Build history of the part. All positions in model axes, mm. A direction names the side the tool comes from. Round coordinates to 2 decimals unless told otherwise and drop trailing zeros. Order: outer loops, then holes, each group sorted by start corner. A loop starts at its lowest first (then second) coordinate and runs counter-clockwise, first axis right, second up. Notation, with made-up numbers: M 80.25,29 L 117.25,29 A14 cw 117.25,42 Z; hole C 61.25,12 d6. An arc over 180 degrees is marked long. One line per item, written item: value. Start each with the question number.
Item 1: Two-plate mould, pull along Z, no slides. Class faces 1 (the flat face through (-1, 15, -24)), 2 (the flat face through (-45, 14, 0.75)), 3 (the flat face through (49, 15, 0)), 4 (the flat face through (-1, 15, 24)): +Z half, -Z half, draft (parallel to the pull), parting line (faces both ways), or undercut.
Item 2: Probe L1, parallel to Z at x = 44, y = 13.25; L2, parallel to X at y = 9.25, z = 20; L3, parallel to X at y = 24, z = 0. List the from-to ranges inside material, lowest first.
Item 3: Tool access for faces 5 (the flat face through (-1, 16, 22.5)), 6 (the flat face through (-49, 15, 0)): list every direction of +Z, -Z, +X, -X, +Y, -Y with a clear straight run to the whole face (end or side of a thin tool).
Item 4: Band-saw the part on C-C, the plane x = -1. Write the cut outline in (y, z).
Item 5: Pin check, flat tips, straight feed: pin 1 (13.5 mm diameter, centred on x = 18.5, z = 1, fed in from +Y); pin 2 (1 mm diameter, centred on x = -10.5, z = -0.5, fed in from -Y); pin 3 (0.8 mm diameter, centred on x = 21, z = -21, fed in from +Y). Stop position of each tip, or through.
Item 6: Band-saw the part on A-A, the plane z = 19. Write the cut outline in (x, y).
```python
from build123d import *

# Parameters (mm, degrees)
SKETCH1_W           = 98
SKETCH1_H           = 48
BOSS_EXTRUDE1_DEPTH = 30
SHELL1_T            = -1.5
SKETCH2_W           = 1.5
SKETCH2_H           = 5
SKETCH2_W_2         = 5
SKETCH2_H_2         = 1.5
BOSS_EXTRUDE2_DEPTH = 25.5


with BuildPart() as part:
    # Sketch1 → Boss-Extrude1 (new body)
    with BuildSketch(Plane(origin=(0, 0, 0), x_dir=(1, 0, 0), z_dir=(0, 1, 0))):
        Rectangle(SKETCH1_W, SKETCH1_H)
    extrude(amount=BOSS_EXTRUDE1_DEPTH)

    # Shell1
    shell1_openings = [part.faces().sort_by_distance(p)[0] for p in [
        (0, 30, 0),
    ]]
    offset(amount=SHELL1_T, openings=shell1_openings, kind=Kind.INTERSECTION)

    # Sketch2 → Boss-Extrude2 (add)
    with BuildSketch(Plane(origin=(0, 1.5, 0), x_dir=(1, 0, 0), z_dir=(0, 1, 0))):
        with Locations((-20.75, 20)):
            Rectangle(SKETCH2_W, SKETCH2_H)
        with Locations((20.75, 20)):
            Rectangle(SKETCH2_W, SKETCH2_H)
        with Locations((20.75, -20)):
            Rectangle(SKETCH2_W, SKETCH2_H)
        with Locations((-20.75, -20)):
            Rectangle(SKETCH2_W, SKETCH2_H)
        with Locations((45, 0)):
            Rectangle(SKETCH2_W_2, SKETCH2_H_2)
        with Locations((-45, 0)):
            Rectangle(SKETCH2_W_2, SKETCH2_H_2)
    extrude(amount=BOSS_EXTRUDE2_DEPTH)


solid = part.part
```
Output:
1. face 1: -Z half
1. face 2: undercut
1. face 3: draft
1. face 4: +Z half
2. L1: z = -24 to -22.5, -0.75 to 0.75, 22.5 to 24
2. L2: x = -49 to -47.5, -21.5 to -20, 20 to 21.5, 47.5 to 49
2. L3: x = -49 to -42.5, 42.5 to 49
3. face 5: +Y
3. face 6: +Z, -Z, -X, +Y, -Y
4. outline: M 0,-24 L 30,-24 L 30,-22.5 L 1.5,-22.5 L 1.5,22.5 L 30,22.5 L 30,24 L 0,24 Z
5. pin 1: stops at y = 1.5
5. pin 2: stops at y = 0
5. pin 3: stops at y = 27
6. outline: M -49,0 L 49,0 L 49,30 L 47.5,30 L 47.5,1.5 L 21.5,1.5 L 21.5,27 L 20,27 L 20,1.5 L -20,1.5 L -20,27 L -21.5,27 L -21.5,1.5 L -47.5,1.5 L -47.5,30 L -49,30 Z
